Can you work these out from the model? Positions are in its coordinate system, mm. A direction names the side the tool comes from. Give positions to 0.01 mm unless a question says otherwise; leave off trailing zeros. Write each loop counter-clockwise with the first axis right and the second up, starting at its lowest first coordinate (ties: lowest second). Pieces come first, ordered by that corner, then holes.
```python
from build123d import *

# Parameters (mm, degrees)
ESQUISSE1_W                = 75
ESQUISSE1_H                = 18.5
BOSS_EXTRU_1_DEPTH         = 7
ENL_V_MAT_EXTRU_1_REACH    = 9
ESQUISSE2_R                = 2
ESQUISSE3_W                = 1.5
ESQUISSE3_H                = 21.5
BOSS_EXTRU_2_DEPTH         = 13
CONG_1_R                   = 4
ESQUISSE4_R                = 1
ENL_V_MAT_EXTRU_2_DEPTH    = 18.5
R_P_TITION_LIN_AIRE1_COUNT = 6
R_P_TITION_LIN_AIRE1_PITCH = 9.65


with BuildPart() as part:
    # Esquisse1 → Boss.-Extru.1 (new body)
    with BuildSketch(Plane.XY):
        with Locations((8.254716981, 3.839622642)):
            Rectangle(ESQUISSE1_W, ESQUISSE1_H)
    extrude(amount=BOSS_EXTRU_1_DEPTH)

    # Esquisse2 → Enlèv. mat.-Extru.1 (cut, up to next)
    with BuildSketch(Plane(origin=(0, 0, 0), x_dir=(-1, 0, 0), z_dir=(0, 0, -1)), mode=Mode.PRIVATE) as enl_v_mat_extru_1_sk1:
        with Locations((-41.754716981, 7.839622642)):
            Circle(ESQUISSE2_R)
    enl_v_mat_extru_1_tool1 = extrude(enl_v_mat_extru_1_sk1.sketch, amount=-ENL_V_MAT_EXTRU_1_REACH, mode=Mode.PRIVATE) & part.part
    add(enl_v_mat_extru_1_tool1.solids().sort_by_distance((41.754717, 7.839623, 0))[0], mode=Mode.SUBTRACT)
    # Esquisse2 → Enlèv. mat.-Extru.1 (cut, up to next)
    with BuildSketch(Plane(origin=(0, 0, 0), x_dir=(-1, 0, 0), z_dir=(0, 0, -1)), mode=Mode.PRIVATE) as enl_v_mat_extru_1_sk2:
        with Locations((-41.754716981, -0.160377358)):
            Circle(ESQUISSE2_R)
    enl_v_mat_extru_1_tool2 = extrude(enl_v_mat_extru_1_sk2.sketch, amount=-ENL_V_MAT_EXTRU_1_REACH, mode=Mode.PRIVATE) & part.part
    add(enl_v_mat_extru_1_tool2.solids().sort_by_distance((41.754717, -0.160377, 0))[0], mode=Mode.SUBTRACT)
    # Esquisse2 → Enlèv. mat.-Extru.1 (cut, up to next)
    with BuildSketch(Plane(origin=(0, 0, 0), x_dir=(-1, 0, 0), z_dir=(0, 0, -1)), mode=Mode.PRIVATE) as enl_v_mat_extru_1_sk3:
        with Locations((25.245283019, -0.160377358)):
            Circle(ESQUISSE2_R)
    enl_v_mat_extru_1_tool3 = extrude(enl_v_mat_extru_1_sk3.sketch, amount=-ENL_V_MAT_EXTRU_1_REACH, mode=Mode.PRIVATE) & part.part
    add(enl_v_mat_extru_1_tool3.solids().sort_by_distance((-25.245283, -0.160377, 0))[0], mode=Mode.SUBTRACT)
    # Esquisse2 → Enlèv. mat.-Extru.1 (cut, up to next)
    with BuildSketch(Plane(origin=(0, 0, 0), x_dir=(-1, 0, 0), z_dir=(0, 0, -1)), mode=Mode.PRIVATE) as enl_v_mat_extru_1_sk4:
        with Locations((25.245283019, 7.839622642)):
            Circle(ESQUISSE2_R)
    enl_v_mat_extru_1_tool4 = extrude(enl_v_mat_extru_1_sk4.sketch, amount=-ENL_V_MAT_EXTRU_1_REACH, mode=Mode.PRIVATE) & part.part
    add(enl_v_mat_extru_1_tool4.solids().sort_by_distance((-25.245283, 7.839623, 0))[0], mode=Mode.SUBTRACT)

    # Esquisse3 → Boss.-Extru.2 (add)
    with BuildSketch(Plane(origin=(0, 0, 0), x_dir=(-1, 0, 0), z_dir=(0, 0, -1))):
        with Locations((-37.504716981, 3.839622642)):
            Rectangle(ESQUISSE3_W, ESQUISSE3_H)
        with Locations((-27.754716981, 3.839622642)):
            Rectangle(ESQUISSE3_W, ESQUISSE3_H)
        with Locations((-18.004716981, 3.839622642)):
            Rectangle(ESQUISSE3_W, ESQUISSE3_H)
        with Locations((-8.254716981, 3.839622642)):
            Rectangle(ESQUISSE3_W, ESQUISSE3_H)
        with Locations((1.495283019, 3.839622642)):
            Rectangle(ESQUISSE3_W, ESQUISSE3_H)
        with Locations((11.245283019, 3.839622642)):
            Rectangle(ESQUISSE3_W, ESQUISSE3_H)
        with Locations((20.995283019, 3.839622642)):
            Rectangle(ESQUISSE3_W, ESQUISSE3_H)
    extrude(amount=-BOSS_EXTRU_2_DEPTH)

    # Congé1
    cong_1_edges = [part.edges().sort_by_distance(p)[0] for p in [
        (8.254716981, -6.910377358, 13),
        (8.254716981, 14.589622642, 13),
        (-1.495283019, -6.910377358, 13),
        (-1.495283019, 14.589622642, 13),
        (-11.245283019, -6.910377358, 13),
        (-11.245283019, 14.589622642, 13),
        (-20.995283019, -6.910377358, 13),
        (-20.995283019, 14.589622642, 13),
        (37.504716981, 14.589622642, 13),
        (37.504716981, -6.910377358, 13),
        (27.754716981, -6.910377358, 13),
        (27.754716981, 14.589622642, 13),
        (18.004716981, -6.910377358, 13),
        (18.004716981, 14.589622642, 13),
    ]]
    fillet(cong_1_edges, radius=CONG_1_R)

    # Esquisse4 → Enlèv. mat.-Extru.2 (cut)
    with BuildSketch(Plane.XZ.offset(5.410377358)):
        with Locations((32.629716981, 7)):
            Circle(ESQUISSE4_R)
    enl_v_mat_extru_2 = extrude(amount=-ENL_V_MAT_EXTRU_2_DEPTH, mode=Mode.SUBTRACT)

    # Répétition linéaire1: Enlèv. mat.-Extru.2 ×6
    with Locations(*[(-i * R_P_TITION_LIN_AIRE1_PITCH, 0, 0) for i in range(1, R_P_TITION_LIN_AIRE1_COUNT)]):
        add(enl_v_mat_extru_2, mode=Mode.SUBTRACT)


solid = part.part
```
1) For faces 4 (the face through (3, -5.41, 3)), 5 (the face through (25, 4, 7)), 6 (the face through (-26, 4, 7)), which set-ups out of +Z, -Z, +X, -X, +Y, -Y let a thin tool reach every point of the face, with its end or its side?
Values follow:
face 4: +Z, -Z, -Y
face 5: +Z, +Y, -Y
face 6: +Z, -X, +Y, -Y
2) Please list where these lines run through material, in increasing order: L1, parallel to X at y = 8, z = 2; L2, parallel to Z at x = -18.5, y = -4; L3, parallel to Y at x = 34, z = 6.
Values follow:
L1: x = -29.25 to -27.24, -23.25 to 39.76, 43.75 to 45.75
L2: z = 0 to 7
L3: y = -5.41 to 13.09
3) Suppose I cut it at C-C on y = 0.75. State how many separate pieces and enclosed holes the cut face has, plus the area to 3 significant figures.
Values follow:
separate pieces: 3
enclosed holes: 0
area: 529 mm2
4) Suppose I cut it at A-A on z = 8. Write out the boundary of the cut face in (x, y), plus the area to 3 significant figures.
Values follow:
outline: (-21.75, -6.91) - (-20.25, -6.91) - (-20.25, 14.59) - (-21.75, 14.59) - close; (-12, -6.91) - (-10.5, -6.91) - (-10.5, 14.59) - (-12, 14.59) - close; (-2.25, -6.91) - (-0.75, -6.91) - (-0.75, 14.59) - (-2.25, 14.59) - close; (7.5, -6.91) - (9, -6.91) - (9, 14.59) - (7.5, 14.59) - close; (17.25, -6.91) - (18.75, -6.91) - (18.75, 14.59) - (17.25, 14.59) - close; (27, -6.91) - (28.5, -6.91) - (28.5, 14.59) - (27, 14.59) - close; (36.75, -6.91) - (38.25, -6.91) - (38.25, 14.59) - (36.75, 14.59) - close
area: 226 mm2
5) Suppose I cut it at B-B on x = 15. Write out the boundary of the cut face in (y, z), plus the area to 4 significant figures.
Values follow:
outline: (-5.41, 0) - (13.09, 0) - (13.09, 7) - (-5.41, 7) - close
area: 129.5 mm2
6) Suppose I cut it at D-D on z = 11.25. Write out the boundary of the cut face in (x, y).
Values follow:
outline: (-21.75, -6.22) - (-20.25, -6.22) - (-20.25, 13.9) - (-21.75, 13.9) - close; (-12, -6.22) - (-10.5, -6.22) - (-10.5, 13.9) - (-12, 13.9) - close; (-2.25, -6.22) - (-0.75, -6.22) - (-0.75, 13.9) - (-2.25, 13.9) - close; (7.5, -6.22) - (9, -6.22) - (9, 13.9) - (7.5, 13.9) - close; (17.25, -6.22) - (18.75, -6.22) - (18.75, 13.9) - (17.25, 13.9) - close; (27, -6.22) - (28.5, -6.22) - (28.5, 13.9) - (27, 13.9) - close; (36.75, -6.22) - (38.25, -6.22) - (38.25, 13.9) - (36.75, 13.9) - close
7) For pin 1 Ø5.5 at (x, z) = (21, 3.5) entering from -Y; pin 2 Ø5 at (x, y) = (41.75, -0.16) entering from +Z; pin 3 Ø2 at (x, z) = (41, 5) entering from -Y; pin 4 Ø1.5 at (y, z) = (2.5, 9.5) entering from -X, each with a flat end and sliding along its axis, tell me the tip position at first contact or that it passes through.
Values follow:
pin 1: stops at y = -6.91
pin 2: stops at z = 7
pin 3: stops at y = -5.41
pin 4: stops at x = -21.75
8) If we mould it in two halves opening along X, with no side actions, what happens to faces 1 (the face through (28.505, 4, 8)), 2 (the face through (42, 4, 7)), 3 (the face through (45.755, 4, 3))? For each: +X half, -X half, draft (parallel to the pull), parting line (faces both ways), or undercut.
Values follow:
face 1: undercut
face 2: draft
face 3: +X half
